Geometry check sheet. Reference: the model listing, model coordinates, mm. A direction names the side the tool comes from. Round coordinates to 2 decimals unless told otherwise and drop trailing zeros. Write each loop counter-clockwise with the first axis right and the second up, starting at its lowest first coordinate (ties: lowest second). Pieces come first, ordered by that corner, then holes. Notation, with made-up numbers: M 2.5,24 L 48.5,24 A20 ccw 48.5,60 Z; hole C 35,62.5 d5. An arc over 180 degrees is marked long. Put each result on its own line as item: value. Start each with the question number.
(1) Mould release check, pull along Z, two halves, no side actions. Record for faces 4 (the flat face through (-47.043, 63.207, 26.628)), 5 (the cylindrical face through (-2.5, 25.9, 43.7)), 6 (the flat face through (-47.043, 63.761, -26.075)): pulls with the +Z half, pulls with the -Z half, needs draft (parallel to the pull), parting line crosses it, or undercut.
(2) Tool access check on faces 1 (the flat face through (7.62, -10, 0)), 2 (the flat face through (-47.043, -54.664, 41.425)), 3 (the cylindrical face through (-25.3, -24.32, 58.66)). Record the directions out of +Z, -Z, +X, -X, +Y, -Y that give a thin tool (end or side, any length) a straight path to the whole face; none if there is none.
(3) Section check A-A on z = 0. Count the separate pieces of the cut face and the enclosed holes in it, then the cut area to 3 significant figures.
(4) Section check B-B on x = -25.5. Record the cut outline in (y, z), then the cut area to 3 significant figures.
(5) Section check D-D on x = -46.5. Record the cut outline in (y, z).
(6) Gauge pin test, flat ends, axial feed: pin 1 (1 mm diameter, centred on x = -44, z = 10, fed in from +Y); pin 2 (1.5 mm diameter, centred on y = -47, z = 44.5, fed in from +X); pin 3 (10 mm diameter, centred on x = -21, z = 29.5, fed in from -Y). Record the tip position at first contact, or that the pin passes through.
(7) Material ranges on probe 1 along Y at (x, z) = (-46, 0); probe 2 along Y at (x, z) = (-22, 0), recorded low to high.
from build123d import *

# Parameters (mm, degrees)
SKETCH3_R           = 25.4
SKETCH1_R           = 50.8
SKETCH4_R           = 63.5
BOSS_EXTRUDE1_DEPTH = 50.8
SHELL1_T            = -5.08
CUT_EXTRUDE1_DEPTH  = 50.8
SKETCH6_R           = 4.826
BOSS_EXTRUDE3_DEPTH = 7.62
FILLET1_R           = 0.508
SKETCH7_R           = 9.525
CUT_EXTRUDE2_DEPTH  = 124.861079859
CIRPATTERN2_COUNT   = 3


with BuildPart() as part:
    # Sketch3 → Loft1 section 0
    with BuildSketch(Plane(origin=(12.7, 0, 0), x_dir=(0, 0, -1), z_dir=(1, 0, 0))):
        Circle(SKETCH3_R)
    # Sketch1 → Loft1 section 1
    with BuildSketch(Plane(origin=(0, 0, 0), x_dir=(0, 0, -1), z_dir=(1, 0, 0))):
        Circle(SKETCH1_R)
    loft()

    # Sketch4 → Boss-Extrude1 (add)
    with BuildSketch(Plane.ZY):
        Circle(SKETCH4_R)
    extrude(amount=BOSS_EXTRUDE1_DEPTH)

    # Shell1
    shell1_openings = [part.faces().sort_by_distance(p)[0] for p in [
        (-50.8, 0, 0),
    ]]
    offset(amount=SHELL1_T, openings=shell1_openings, kind=Kind.INTERSECTION)

    # Sketch5 → Cut-Extrude1 (cut)
    with BuildSketch(Plane(origin=(12.7, 0, 0), x_dir=(0, 0, -1), z_dir=(1, 0, 0))):
        with BuildLine():
            Line((-12.7, 21.997045256), (-12.7, 49.186888497))
            ThreePointArc((-12.7, 49.186888497), (-43.994090512, 25.4), (-48.947094971, -13.59492162))
            Line((-48.947094971, -13.59492162), (-25.4, 0))
            ThreePointArc((-25.4, 0), (-21.997045256, 12.7), (-12.7, 21.997045256))
        make_face()
        with BuildLine():
            Line((12.7, 21.997045256), (12.7, 49.186888497))
            ThreePointArc((12.7, 49.186888497), (43.994090512, 25.4), (48.947094971, -13.59492162))
            Line((48.947094971, -13.59492162), (25.4, 0))
            ThreePointArc((25.4, 0), (21.997045256, 12.7), (12.7, 21.997045256))
        make_face()
        with BuildLine():
            Line((12.7, -21.997045256), (36.247094971, -35.591966876))
            ThreePointArc((36.247094971, -35.591966876), (0, -50.8), (-36.247094971, -35.591966876))
            Line((-36.247094971, -35.591966876), (-12.7, -21.997045256))
            ThreePointArc((-12.7, -21.997045256), (0, -25.4), (12.7, -21.997045256))
        make_face()
    extrude(amount=-CUT_EXTRUDE1_DEPTH, mode=Mode.SUBTRACT)

    # Sketch6 → Boss-Extrude3 (add)
    with BuildSketch(Plane.ZY.offset(50.8)):
        with BuildLine():
            ThreePointArc((7.762367521, 82.105471512), (0.023010453, 85.305702571), (-7.729809299, 82.138225256))
            Line((-7.729809299, 82.138225256), (-44.940751738, 44.861774744))
            ThreePointArc((-44.940751738, 44.861774744), (0, 63.5), (44.940751738, 44.861774744))
            Line((44.940751738, 44.861774744), (7.79520225, 82.072717183))
            ThreePointArc((7.79520225, 82.072717183), (7.778802125, 82.089111629), (7.762367521, 82.105471512))
        make_face()
        with Locations((0, 74.422)):
            Circle(SKETCH6_R, mode=Mode.SUBTRACT)
    boss_extrude3 = extrude(amount=-BOSS_EXTRUDE3_DEPTH)

    # Fillet1
    fillet1_edges = [part.edges().sort_by_distance(p)[0] for p in [
        (0, 0, -63.5),
    ]]
    fillet(fillet1_edges, radius=FILLET1_R)

    # Sketch7 → Cut-Extrude2 (cut, through all)
    with BuildSketch(Plane(origin=(12.7, 0, 0), x_dir=(0, 0, -1), z_dir=(1, 0, 0))):
        Circle(SKETCH7_R)
    extrude(amount=-CUT_EXTRUDE2_DEPTH, mode=Mode.SUBTRACT)

    # CirPattern2: Boss-Extrude3 ×3 about axis
    cirpattern2_axis = Axis((0, 0, 0), (1, 0, 0))
    for i in range(1, CIRPATTERN2_COUNT):
        add(boss_extrude3.rotate(cirpattern2_axis, i * 360 / CIRPATTERN2_COUNT))


solid = part.part
Answers follow:
1. face 4: pulls with the +Z half
1. face 5: undercut
1. face 6: pulls with the -Z half
2. face 1: -X
2. face 2: +Z, +X, -X, -Y
2. face 3: +X
3. separate pieces: 4
3. enclosed holes: 0
3. area: 992 mm^2
4. outline: C 0,0 d127; hole C 0,0 d116.84
4. area: 1,950 mm^2
5. outline: M -61.35,-16.38 L -47.76,-67.27 A11.01 ccw -34.33,-74.99 A11.01 ccw -34.29,-74.97 L 16.49,-61.32 A63.5 ccw 44.86,-44.94 L 82.14,-7.73 A11.01 ccw 82.11,7.76 A11.01 ccw 82.07,7.8 L 44.86,44.94 A63.5 ccw 16.49,61.32 L -34.37,75 A11.01 ccw -47.78,67.22 A11.01 ccw -47.79,67.18 L -61.35,16.38 A63.5 ccw Z; hole C 0,0 d116.84; hole C -37.21,-64.45 d9.65; hole C -37.21,64.45 d9.65; hole C 74.42,0 d9.65
6. pin 1: stops at y = 80.36
6. pin 2: stops at x = -43.18
6. pin 3: stops at y = -58.58
7. probe 1: y = -63.5 to -58.42, 58.42 to 69.6, 79.25 to 85.31
7. probe 2: y = -63.5 to -58.42, 58.42 to 63.5
